from build123d import *

# Parameters (mm, degrees)
F1_DEPTH = 50
F2_R     = 5.5
F3_DEPTH = 5
F4_R     = 3.1
F5_DEPTH = 5.001


with BuildPart() as f1:
    # F0 (on Front) → F1 (new body, symmetric)
    with BuildSketch(Plane.XZ):
        Polygon((16.613249, -2.5), (19.5, -2.5), (19.5, 2.5), (-19.5, 2.5), (-19.5, -2.5), (-16.613249, -2.5), (-19.5, -7.5), (19.5, -7.5), align=None)
    extrude(amount=F1_DEPTH, both=True)

    # F2 (on face) → F3 (cut)
    with BuildSketch(Plane(origin=(0, 0, -7.5), x_dir=(1, 0, 0), z_dir=(0, 0, -1))):
        Circle(F2_R)
        with Locations((0, -42)):
            Circle(F2_R)
        with Locations((0, 42)):
            Circle(F2_R)
        with BuildLine():
            ThreePointArc((-5.5, -30), (0, -35.5), (5.5, -30))
            ThreePointArc((5.5, -30), (0, -24.5), (-5.5, -30))
        make_face()
        with BuildLine():
            ThreePointArc((-5.5, -30), (0, -24.5), (5.5, -30))
            Line((5.5, -30), (5.5, -12))
            ThreePointArc((5.5, -12), (0, -17.5), (-5.5, -12))
            Line((-5.5, -12), (-5.5, -30))
        make_face()
        with BuildLine():
            ThreePointArc((-5.5, -12), (0, -17.5), (5.5, -12))
            ThreePointArc((5.5, -12), (0, -6.5), (-5.5, -12))
        make_face()
        with BuildLine():
            ThreePointArc((-5.5, 12), (0, 6.5), (5.5, 12))
            ThreePointArc((5.5, 12), (0, 17.5), (-5.5, 12))
        make_face()
        with BuildLine():
            ThreePointArc((-5.5, 12), (0, 17.5), (5.5, 12))
            Line((5.5, 12), (5.5, 30))
            ThreePointArc((5.5, 30), (0, 24.5), (-5.5, 30))
            Line((-5.5, 30), (-5.5, 12))
        make_face()
        with BuildLine():
            ThreePointArc((-5.5, 30), (0, 24.5), (5.5, 30))
            ThreePointArc((5.5, 30), (0, 35.5), (-5.5, 30))
        make_face()
    extrude(amount=-F3_DEPTH, mode=Mode.SUBTRACT)

    # F4 (on face) → F5 (cut, through all)
    with BuildSketch(Plane(origin=(0, 0, -2.5), x_dir=(1, 0, 0), z_dir=(0, 0, -1))):
        with Locations((0, -42)):
            Circle(F4_R)
        Circle(F4_R)
        with Locations((0, 42)):
            Circle(F4_R)
        with BuildLine():
            ThreePointArc((-3.1, -30), (0, -33.1), (3.1, -30))
            ThreePointArc((3.1, -30), (0, -26.9), (-3.1, -30))
        make_face()
        with BuildLine():
            ThreePointArc((-3.1, -30), (0, -26.9), (3.1, -30))
            Line((3.1, -30), (3.1, -12))
            ThreePointArc((3.1, -12), (0, -15.1), (-3.1, -12))
            Line((-3.1, -12), (-3.1, -30))
        make_face()
        with BuildLine():
            ThreePointArc((-3.1, -12), (0, -15.1), (3.1, -12))
            ThreePointArc((3.1, -12), (0, -8.9), (-3.1, -12))
        make_face()
        with BuildLine():
            ThreePointArc((-3.1, 12), (0, 8.9), (3.1, 12))
            ThreePointArc((3.1, 12), (0, 15.1), (-3.1, 12))
        make_face()
        with BuildLine():
            ThreePointArc((-3.1, 12), (0, 15.1), (3.1, 12))
            Line((3.1, 12), (3.1, 30))
            ThreePointArc((3.1, 30), (0, 26.9), (-3.1, 30))
            Line((-3.1, 30), (-3.1, 12))
        make_face()
        with BuildLine():
            ThreePointArc((-3.1, 30), (0, 26.9), (3.1, 30))
            ThreePointArc((3.1, 30), (0, 33.1), (-3.1, 30))
        make_face()
    extrude(amount=-F5_DEPTH, mode=Mode.SUBTRACT)


solid = f1.part
Model file for the job. Use its own axes, mm. A direction names the side the tool comes from. Round coordinates to 2 decimals unless told otherwise and drop trailing zeros. Loops run counter-clockwise (first coordinate to the right, second up) from the corner with the lowest first, then second, coordinate; pieces in that order, holes last.
1. Wall check: probe 1 along Y at (x, z) = (0, -6.05); probe 2 along Y at (x, z) = (0, 1.4); probe 3 along X at (y, z) = (42, 0.9). Give the ranges that are in metal, low to high.
Check values:
probe 1: y = -50 to -47.5, -36.5 to -35.5, -6.5 to -5.5, 5.5 to 6.5, 35.5 to 36.5, 47.5 to 50
probe 2: y = -50 to -45.1, -38.9 to -33.1, -8.9 to -3.1, 3.1 to 8.9, 33.1 to 38.9, 45.1 to 50
probe 3: x = -19.5 to -3.1, 3.1 to 19.5
2. Band-saw the part on C-C, the plane x = 4. List the corners of the cut face in (y, z).
Check values:
outline: (-50, -7.5) - (-45.77, -7.5) - (-45.77, -2.5) - (-38.23, -2.5) - (-38.23, -7.5) - (-33.77, -7.5) - (-33.77, -2.5) - (-8.23, -2.5) - (-8.23, -7.5) - (-3.77, -7.5) - (-3.77, -2.5) - (3.77, -2.5) - (3.77, -7.5) - (8.23, -7.5) - (8.23, -2.5) - (33.77, -2.5) - (33.77, -7.5) - (38.23, -7.5) - (38.23, -2.5) - (45.77, -2.5) - (45.77, -7.5) - (50, -7.5) - (50, 2.5) - (-50, 2.5) - close
3. Tool access for faces 1 (the cylindrical face through (-0.1, 35.5, -5)), 2 (the cylindrical face through (-0.1, 33.1, 0)), 3 (the flat face through (-9, -1, -7.5)): list every direction of +Z, -Z, +X, -X, +Y, -Y with a clear straight run to the whole face (end or side of a thin tool).
Check values:
face 1: -Z
face 2: +Z, -Z
face 3: -Z, +X, -X, +Y, -Y
4. Band-saw the part on A-A, the plane y = 42. List the corners of the cut face in (x, z).
Check values:
outline: (-19.5, -7.5) - (-5.5, -7.5) - (-5.5, -2.5) - (-3.1, -2.5) - (-3.1, 2.5) - (-19.5, 2.5) - (-19.5, -2.5) - (-16.61, -2.5) - close; (3.1, -2.5) - (5.5, -2.5) - (5.5, -7.5) - (19.5, -7.5) - (16.61, -2.5) - (19.5, -2.5) - (19.5, 2.5) - (3.1, 2.5) - close
5. Mould opens along X. For faces 4 (the flat face through (19.5, -1, 0)), 5 (the flat face through (-5.5, 21, -5)), 6 (the flat face through (-18.04, -0.7, -4.97)) say: +X half, -X half, draft (parallel to the pull), parting line (faces both ways), or undercut.
Check values:
face 4: +X half
face 5: undercut
face 6: -X half
6. Drop flat-ended pins along their axis: P1, Ø4, axis at y = -22.5, z = -5, coming from the -X side; P2, Ø12, axis at x = 2, y = 2, coming from the -Z side; P3, Ø5.5, axis at x = -2.5, y = 20, coming from the -Z side; P4, Ø2.5, axis at y = 22, z = -5.5, coming from the +X side. Give the stop position or say it passes through.
Check values:
P1: stops at x = -19.21
P2: stops at z = -7.5
P3: stops at z = -2.5
P4: stops at x = 19.07
7. Band-saw the part on B-B, the plane z = -1.25. List the corners of the cut face in (x, y).
Check values:
outline: (-19.5, -50) - (19.5, -50) - (19.5, 50) - (-19.5, 50) - close; hole circle Ø6.2 at (0, -42); hole (-3.1, -30) arc R3.1 ccw to (3.1, -30) - (3.1, -12) arc R3.1 ccw to (-3.1, -12) - close; hole circle Ø6.2 at (0, 0); hole (-3.1, 12) arc R3.1 ccw to (3.1, 12) - (3.1, 30) arc R3.1 ccw to (-3.1, 30) - close; hole circle Ø6.2 at (0, 42)
